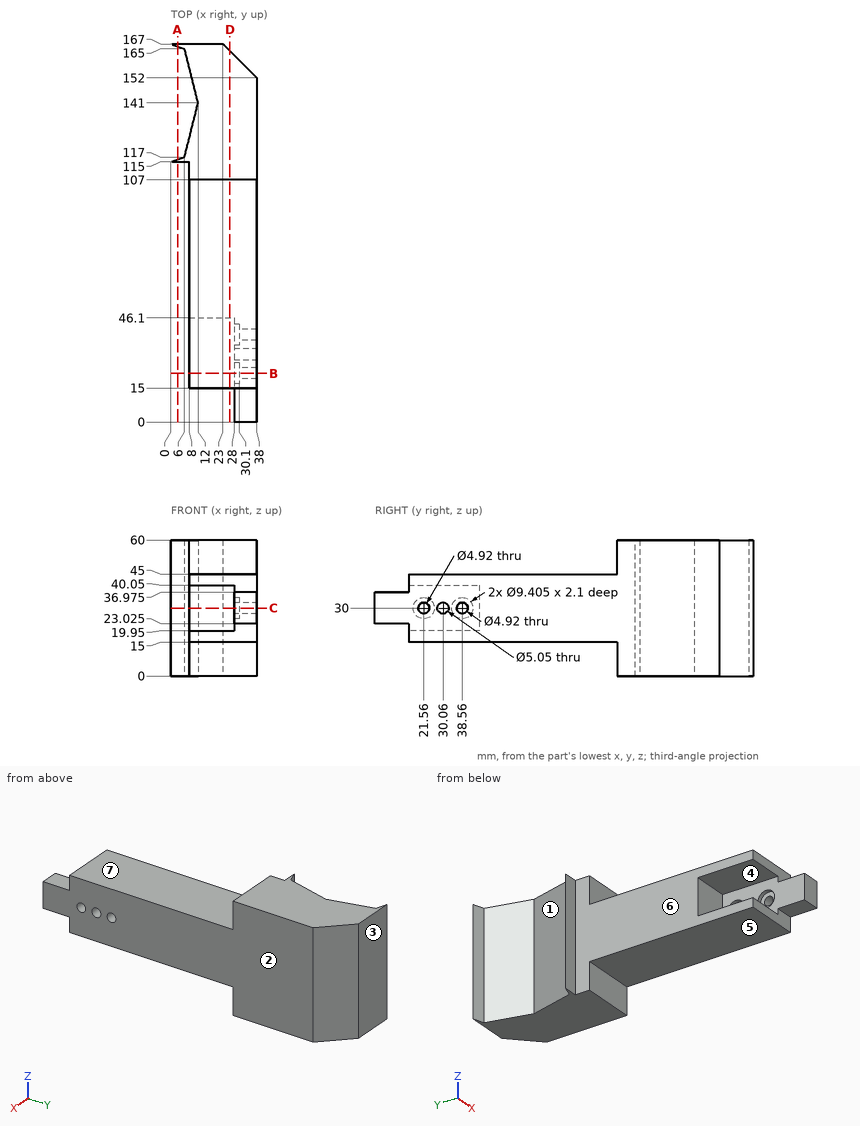
Source: three-view drawing plus pictorial views. Frame: mm from the lowest corner of the part. A direction names the side the tool comes from. Round coordinates to 2 decimals unless told otherwise and drop trailing zeros. Loops run counter-clockwise (first coordinate to the right, second up) from the corner with the lowest first, then second, coordinate; pieces in that order, holes last.
Item 1: Section B-B, the plane y = 21.56. Output: boundary loops of the cut face in (x, z), plus the area to 3 significant figures.
Checked values:
outline: (8, 15) - (38, 15) - (38, 27.54) - (30.1, 27.54) - (30.1, 25.3) - (28, 25.3) - (28, 19.95) - (8, 19.95) - close; (8, 40.05) - (28, 40.05) - (28, 34.7) - (30.1, 34.7) - (30.1, 32.46) - (38, 32.46) - (38, 45) - (8, 45) - close
area: 439 mm2
Item 2: Line query: L1, parallel to Z at x = 35.5, y = 21.56; L2, parallel to Z at x = 12, y = 36.5; L3, parallel to Z at x = 22.5, y = 52. Output: solid intervals per line, ascending.
Checked values:
L1: z = 15 to 27.54, 32.46 to 45
L2: z = 15 to 19.95, 40.05 to 45
L3: z = 15 to 45
Item 3: Section C-C, the plane z = 30. State how many separate pieces and enclosed holes the cut face has, plus the area to 3 significant figures.
Checked values:
separate pieces: 4
enclosed holes: 0
area: 3,780 mm2
Item 4: Reachability of the marked faces 4, 5, 6 and 7 from +Z, -Z, +X, -X, +Y, -Y: full face, straight path, thin tool, end or side. Return the list, or none.
Checked values:
face 4: -X, -Y
face 5: -Z, +X, -X, -Y
face 6: +Z, -Z, -X, -Y
face 7: +Z, +X, -X, -Y
Item 5: Mould query, pull axis Y, two halves, no side actions, for the marked faces 1, 2 and 3. Classes: released by +Y, released by -Y, zero draft, split by the parting line, or undercut.
Checked values:
face 1: undercut
face 2: zero draft
face 3: released by +Y
Item 6: Section D-D, the plane x = 26. Output: boundary loops of the cut face in (y, z).
Checked values:
outline: (15, 15) - (107, 15) - (107, 0) - (164, 0) - (164, 60) - (107, 60) - (107, 45) - (15, 45) - (15, 40.05) - (46.1, 40.05) - (46.1, 19.95) - (15, 19.95) - close
Item 7: Contact query for flat-ended pins moving along their axis: P1, Ø8, axis at y = 21.56, z = 30, coming from the -X side; P2, Ø6, axis at y = 84.5, z = 38.5, coming from the -X side; P3, Ø11, axis at x = 31, y = 4, coming from the -Z side (3 decimals); P4, Ø3, axis at y = 38.56, z = 30, coming from the +X side. Output: stop coordinate, or through.
Checked values:
P1: stops at x = 30.1
P2: stops at x = 8
P3: stops at z = 23.025
P4: passes through
Item 8: Section A-A, the plane x = 3. Output: boundary loops of the cut face in (y, z), plus the area to 3 significant figures.
Checked values:
outline: (115, 0) - (116, 0) - (116, 60) - (115, 60) - close; (166, 0) - (167, 0) - (167, 60) - (166, 60) - close
area: 120 mm2
